Source: CAD feature listing. Evaluate the final solid. Frame: model axes, mm. A direction names the side the tool comes from. Give positions to 0.01 mm unless a question says otherwise; leave off trailing zeros. Order: outer loops, then holes, each group sorted by start corner. A loop starts at its lowest first (then second) coordinate and runs counter-clockwise, first axis right, second up.
from build123d import *

# Parameters (mm, degrees)
BOSS_EXTRUDE1_DEPTH = 10
SKETCH1_4_R         = 11.5
BOSS_EXTRUDE3_DEPTH = 5
BOSS_EXTRUDE4_DEPTH = 5
BOSS_EXTRUDE5_DEPTH = 20
SKETCH1_8_R         = 11.5
SKETCH1_8_R_2       = 8.8
SKETCH1_8_R_3       = 8
BOSS_EXTRUDE6_DEPTH = 5
SKETCH1_10_R        = 8.8
SKETCH1_10_R_2      = 8
BOSS_EXTRUDE8_DEPTH = 20
SKETCH8_R           = 4
CUT_EXTRUDE2_DEPTH  = 20


with BuildPart() as part:
    # Sketch1 → Boss-Extrude1 (new body)
    with BuildSketch(Plane(origin=(0, 0, 0), x_dir=(1, 0, 0), z_dir=(0, 1, 0))):
        with BuildLine():
            Line((-7.705545208, -4.250243881), (-7.005041098, -3.863858073))
            ThreePointArc((-7.005041098, -3.863858073), (-3.863858073, 7.005041098), (7.005041098, 3.863858073))
            Line((7.005041098, 3.863858073), (7.705545208, 4.250243881))
            ThreePointArc((7.705545208, 4.250243881), (-4.250243881, 7.705545208), (-7.705545208, -4.250243881))
        make_face()
    extrude(amount=BOSS_EXTRUDE1_DEPTH)

    # Sketch1<4> → Boss-Extrude3 (add)
    with BuildSketch(Plane(origin=(0, 0, 0), x_dir=(1, 0, 0), z_dir=(0, 1, 0))):
        Circle(SKETCH1_4_R)
        with BuildLine():
            Line((-7.705545208, -4.250243881), (-7.005041098, -3.863858073))
            ThreePointArc((-7.005041098, -3.863858073), (3.863858073, -7.005041098), (7.005041098, 3.863858073))
            Line((7.005041098, 3.863858073), (7.705545208, 4.250243881))
            ThreePointArc((7.705545208, 4.250243881), (4.250243881, -7.705545208), (-7.705545208, -4.250243881))
        make_face(mode=Mode.SUBTRACT)
    extrude(amount=-BOSS_EXTRUDE3_DEPTH)

    # Sketch1<6> → Boss-Extrude4 (add)
    with BuildSketch(Plane(origin=(0, 0, 0), x_dir=(1, 0, 0), z_dir=(0, 1, 0))):
        with BuildLine():
            ThreePointArc((8, 0), (1.994952532, -7.747268189), (-7.005041098, -3.863858073))
            Line((-7.005041098, -3.863858073), (-7.705545208, -4.250243881))
            ThreePointArc((-7.705545208, -4.250243881), (2.194447786, -8.521995008), (8.8, 0))
            ThreePointArc((8.8, 0), (8.521995008, 2.194447786), (7.705545208, 4.250243881))
            Line((7.705545208, 4.250243881), (7.005041098, 3.863858073))
            ThreePointArc((7.005041098, 3.863858073), (7.747268189, 1.994952532), (8, 0))
        make_face()
    extrude(amount=-BOSS_EXTRUDE4_DEPTH)

    # Sketch1<7> → Boss-Extrude5 (add)
    with BuildSketch(Plane(origin=(0, 0, 0), x_dir=(1, 0, 0), z_dir=(0, 1, 0))):
        with BuildLine():
            ThreePointArc((7.005041098, 3.863858073), (-3.863858073, 7.005041098), (-7.005041098, -3.863858073))
            Line((-7.005041098, -3.863858073), (7.005041098, 3.863858073))
        make_face()
    extrude(amount=BOSS_EXTRUDE5_DEPTH)

    # Sketch1<8> → Boss-Extrude6 (add)
    with BuildSketch(Plane(origin=(0, 0, 0), x_dir=(1, 0, 0), z_dir=(0, 1, 0))):
        Circle(SKETCH1_8_R)
        Circle(SKETCH1_8_R_2, mode=Mode.SUBTRACT)
        Circle(SKETCH1_8_R_3)
    extrude(amount=-BOSS_EXTRUDE6_DEPTH)

    # Sketch1<10> → Boss-Extrude8 (add)
    with BuildSketch(Plane(origin=(0, 0, 0), x_dir=(1, 0, 0), z_dir=(0, 1, 0))):
        Circle(SKETCH1_10_R)
        Circle(SKETCH1_10_R_2, mode=Mode.SUBTRACT)
    extrude(amount=-BOSS_EXTRUDE8_DEPTH)

    # Sketch8 → Cut-Extrude2 (cut)
    with BuildSketch(Plane(origin=(0, 0, 0), x_dir=(0.875630137, 0, -0.482982259), z_dir=(0.482982259, 0, 0.875630137))):
        with Locations((0.5, 10)):
            Circle(SKETCH8_R)
    extrude(amount=-CUT_EXTRUDE2_DEPTH, mode=Mode.SUBTRACT)


solid = part.part
(1) Line query: line 1 along X through (y, z) = (-9.5, 0); line 2 along Y through (x, z) = (8.25, -0.75). Output: solid intervals per line, ascending.
(2) Section C-C, the plane z = 7. Return loops of the section in (x, y).
(3) Pin query (flat end, axial travel): pin 1 Ø4 at (y, z) = (12, -7) entering from +X (3 decimals); pin 2 Ø4 at (y, z) = (-15.5, 2.5) entering from -X; pin 3 Ø4 at (x, y) = (-6, -8) entering from -Z. Return the tip coordinate at first contact, or that it passes through.
(4) Section A-A, the plane y = 7. Return loops of the section in (x, z).
(5) Section B-B, the plane y = 18. Return loops of the section in (x, z), plus the area to 3 significant figures.
(6) Draft query along Z for faces 1 (the cylindrical face through (-3.709, 14.93, -7.088)), 2 (the cylindrical face through (-1.73, -12.4, 7.81)), 3 (the flat face through (5, 10, -7)). Return one class per face: +Z half, -Z half, draft (parallel to the pull), parting line (faces both ways), or undercut.
(7) Access query for faces 4 (the flat face through (2, -20, 8)), 5 (the flat face through (6, -5, 7)), 6 (the flat face through (2, 0, 2)), 7 (the flat face through (-8.2, 10, -0.2)). Directions: +Z, -Z, +X, -X, +Y, -Y. A direction counts if a zero-diameter tool reaches every point of the face in a straight line with its end or side. Return the directions, or none.
(8) Section D-D, the plane x = -9.5. Return loops of the section in (y, z).
Checks:
1. line 1: x = -8.8 to -8, 8 to 8.8
1. line 2: y = -20 to 0
2. outline: (-9.12, -5) - (-5.33, -5) - (-5.33, -20) - (-3.87, -20) - (-3.87, -5) - (3.87, -5) - (3.87, -20) - (5.33, -20) - (5.33, -5) - (9.12, -5) - (9.12, 0) - (-9.12, 0) - close
3. pin 1: stops at x = 6.245
3. pin 2: stops at x = -8.79
3. pin 3: stops at z = -7.84
4. outline: (-7.71, 4.25) arc R8.8 ccw to (-6, -6.44) - (-1.88, 1.04) - close; (-1.21, -8.72) arc R8.8 ccw to (7.71, -4.25) - (2.75, -1.52) - close
5. outline: (-7.01, 3.86) arc R8 ccw to (7.01, -3.86) - close
5. area: 101 mm2
6. face 1: parting line
6. face 2: undercut
6. face 3: draft
7. face 4: +Z, -Z, +X, -X, -Y
7. face 5: -Y
7. face 6: +Y
7. face 7: -X, +Y
8. outline: (-5, -6.48) - (0, -6.48) - (0, 6.48) - (-5, 6.48) - close
